Could you check a few things on this drawing? It's one solid part, dimensions in mm from its lowest x, y, z. A direction names the side the tool comes from. Coordinates: 2 decimals unless noted, no trailing zeros. Order: outer loops, then holes, each group sorted by start corner. A loop starts at its lowest first (then second) coordinate and runs counter-clockwise, first axis right, second up.
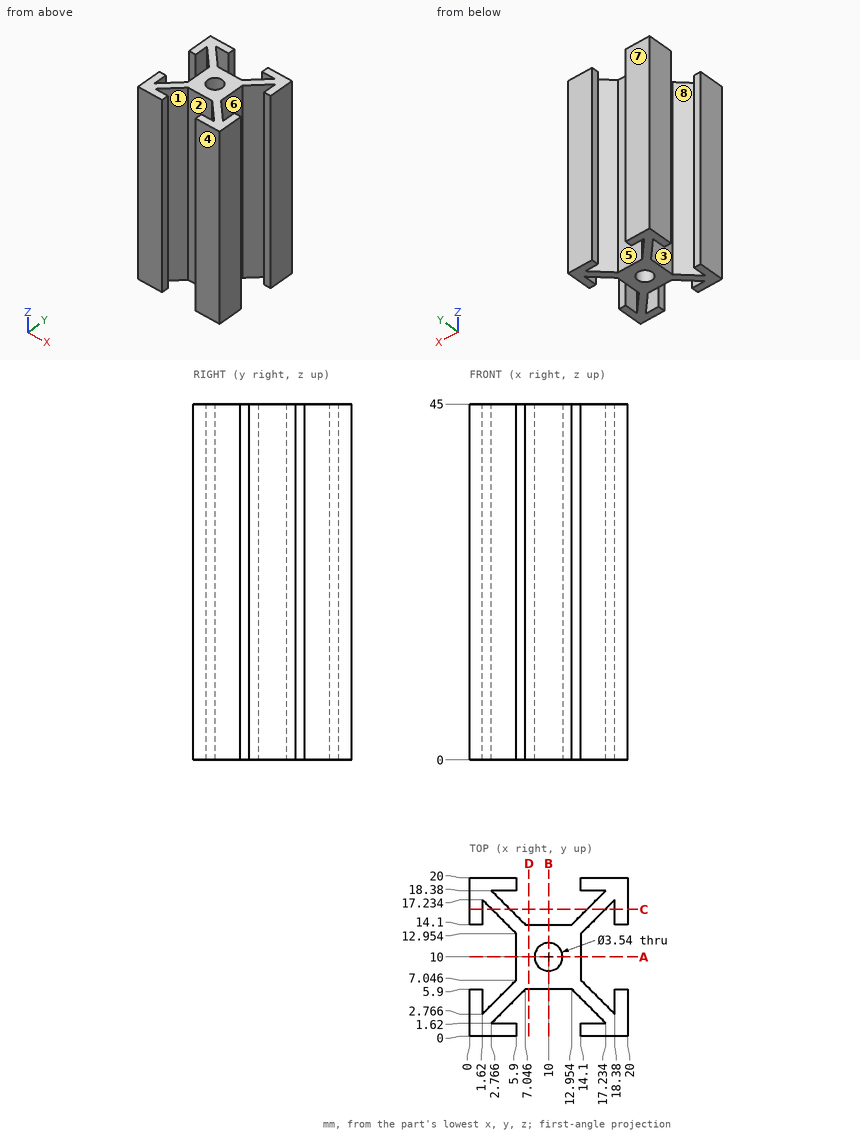
Item 1: Which directions (+Z, -Z, +X, -X, +Y, -Y) give clear straight access to the entire face, cutting with the end or side of a thin tool? Please do the marked faces 1, 2, 3, 4 and 5.
Item 2: Suppose I cut it at D-D (x = 7.5). List the corners of the cut face in (y, z) for me, and give its area (3 significant figures).
Item 3: I need wall thicknesses on line 1 (X direction, y = 10, z = 30); line 2 (Y direction, x = 4.25, z = 43.5) (1 decimal). Which ranges of each line are inside material? Lowest first, please.
Item 4: For pin 1 Ø1.8 at (y, z) = (10, 17) entering from +X; pin 2 Ø1.5 at (x, z) = (12, 30) entering from +Y; pin 3 Ø5 at (x, z) = (11, 38.5) entering from -Y (1 decimal), each with a flat end and sliding along its axis, tell me the tip position at first contact or that it passes through.
Item 5: Suppose I cut it at C-C (y = 16). List the corners of the cut face in (x, z) for me (1 decimal), and give its area (3 significant figures).
Item 6: Suppose I cut it at A-A (y = 10). List the corners of the cut face in (x, z) for me.
Item 7: Thinking about a two-plate mould opening in X: for the marked faces 6, 7 and 8, which applies, +X half, -X half, draft (parallel to the pull), parting line (faces both ways), or undercut?
Geometry results:
1. face 1: +Z, -Z
1. face 2: +Z, -Z, -Y
1. face 3: +Z, -Z, -X
1. face 4: +Z, -Z, +X, -X, -Y
1. face 5: +Z, -Z, +Y
2. outline: (5.9, 0) - (14.1, 0) - (14.1, 45) - (5.9, 45) - close
2. area: 369 mm2
3. line 1: x = 5.9 to 8.23, 11.77 to 14.1
3. line 2: y = 0 to 1.6, 3.1 to 5.4, 14.6 to 16.9, 18.4 to 20
4. pin 1: stops at x = 14.1
4. pin 2: stops at y = 14.1
4. pin 3: stops at y = 5.4
5. outline: (0, 0) - (1.6, 0) - (1.6, 45) - (0, 45) - close; (2.9, 0) - (5.1, 0) - (5.1, 45) - (2.9, 45) - close; (14.9, 0) - (17.1, 0) - (17.1, 45) - (14.9, 45) - close; (18.4, 0) - (20, 0) - (20, 45) - (18.4, 45) - close
5. area: 352 mm2
6. outline: (5.9, 0) - (8.23, 0) - (8.23, 45) - (5.9, 45) - close; (11.77, 0) - (14.1, 0) - (14.1, 45) - (11.77, 45) - close
7. face 6: +X half
7. face 7: draft
7. face 8: undercut
